Read the model definition and answer for the solid it produces. Units are mm, in the model's axes. A direction names the side the tool comes from. Coordinates: 2 decimals unless noted, no trailing zeros. Loops run counter-clockwise (first coordinate to the right, second up) from the corner with the lowest first, then second, coordinate; pieces in that order, holes last. Notation, with made-up numbers: (61, -24) - (104, -24) arc R20 ccw to (104, -17) - close; hole circle Ø8 at (16, -5). An arc over 180 degrees is marked (long way). One line per item, written item: value. Start each with the question number.
from build123d import *

# Parameters (mm, degrees)
EXTRUDE1_DEPTH                                      = 8
CBORE_FOR_M4_HEX_SOCKET_HEAD_CAP_SCREW1_D           = 4.5
CBORE_FOR_M4_HEX_SOCKET_HEAD_CAP_SCREW1_CBORE_D     = 8
CBORE_FOR_M4_HEX_SOCKET_HEAD_CAP_SCREW1_CBORE_DEPTH = 4.4
M5_TAPPED_HOLE1_D                                   = 4.2


with BuildPart() as part:
    # Sketch1 → Extrude1 (new body)
    with BuildSketch(Plane.XY):
        with BuildLine():
            Line((0, 6), (0, 14))
            ThreePointArc((0, 14), (-1.757359313, 18.242640687), (-6, 20))
            Line((-6, 20), (-7, 20))
            ThreePointArc((-7, 20), (-11.242640687, 21.757359313), (-13, 26))
            Line((-13, 26), (-13, 29))
            ThreePointArc((-13, 29), (-11.242640687, 33.242640687), (-7, 35))
            Line((-7, 35), (6, 35))
            ThreePointArc((6, 35), (10.242640687, 33.242640687), (12, 29))
            Line((12, 29), (12, 0))
            Line((12, 0), (6, 0))
            ThreePointArc((6, 0), (1.757359313, 1.757359313), (0, 6))
        make_face()
    extrude(amount=EXTRUDE1_DEPTH)

    # CBORE for M4 Hex Socket Head Cap Screw1 (through all)
    with Locations(Plane.XY.offset(8)):
        with Locations((-6.5, 27.5), (5.5, 27.5)):
            CounterBoreHole(CBORE_FOR_M4_HEX_SOCKET_HEAD_CAP_SCREW1_D / 2, CBORE_FOR_M4_HEX_SOCKET_HEAD_CAP_SCREW1_CBORE_D / 2, CBORE_FOR_M4_HEX_SOCKET_HEAD_CAP_SCREW1_CBORE_DEPTH)

    # M5 Tapped Hole1 (through all)
    with Locations(Plane(origin=(12, 0, 0), x_dir=(0, 0, -1), z_dir=(1, 0, 0))):
        with Locations((-4, 7)):
            Hole(M5_TAPPED_HOLE1_D / 2)


solid = part.part
1) Section C-C, the plane y = 27.5 is taken. Determine the outline of the cut face in (x, z), and give its area (3 significant figures).
2) Determine the mould class of faces 4 (the cylindrical face through (-7.538, 25.504, 1.775)), 5 (the cylindrical face through (-7.021, 31.466, 5.831)), 6 (the flat face through (0, 11, 4)), 7 (the flat face through (9, 0, 4)) for opening direction X: released by +X, released by -X, zero draft, split by the parting line, or undercut.
3) Straight lines are drawn through the part: L1, parallel to X at y = 26, z = 4.5; L2, parallel to Y at x = -6.5, z = 1.3; L3, parallel to Y at x = -6.5, z = 5.2. For each, find the intervals that lie inside material, in ascending order.
4) Section B-B, the plane y = 7 is taken. Determine the outline of the cut face in (x, z).
5) Section D-D, the plane z = 5.25 is taken. Determine the outline of the cut face in (x, y).
6) For faces 1 (the flat face through (12, 15, 4)), 2 (the flat face through (-6.5, 20, 3.9)), 3 (the flat face through (7.2, 25.8, 3.6)), determine the directions among +Z, -Z, +X, -X, +Y, -Y from which every point of the face is accessible in a straight line to the end or side of a thin tool.
7) Flat-ended cylindrical pins translate along their axes: P1, Ø7, axis at x = -6.5, y = 27.5, coming from the +Z side; P2, Ø1.5, axis at x = -5.5, z = 6.5, coming from the -Y side; P3, Ø4, axis at y = 8, z = 2.5, coming from the -X side. Find the tip coordinate at first contact, or state that the pin passes through.
8) Section A-A, the plane x = -6.5 is taken. Determine the outline of the cut face in (y, z).
Answer below:
1. outline: (-13, 0) - (-8.75, 0) - (-8.75, 3.6) - (-10.5, 3.6) - (-10.5, 8) - (-13, 8) - close; (-4.25, 0) - (3.25, 0) - (3.25, 3.6) - (1.5, 3.6) - (1.5, 8) - (-2.5, 8) - (-2.5, 3.6) - (-4.25, 3.6) - close; (7.75, 0) - (12, 0) - (12, 8) - (9.5, 8) - (9.5, 3.6) - (7.75, 3.6) - close
1. area: 97.2 mm2
2. face 4: undercut
2. face 5: undercut
2. face 6: released by -X
2. face 7: zero draft
3. L1: -13 to -10.21, -2.79 to 1.79, 9.21 to 12
3. L2: 20 to 25.25, 29.75 to 35
3. L3: 20 to 23.5, 31.5 to 35
4. outline: (0, 0) - (12, 0) - (12, 1.9) - (0, 1.9) - close; (0, 6.1) - (12, 6.1) - (12, 8) - (0, 8) - close
5. outline: (-13, 26) arc R6 ccw to (-7, 20) - (-6, 20) arc R6 cw to (0, 14) - (0, 8.69) - (12, 8.69) - (12, 29) arc R6 ccw to (6, 35) - (-7, 35) arc R6 ccw to (-13, 29) - close; (0.04, 5.31) arc R6 ccw to (6, 0) - (12, 0) - (12, 5.31) - close; hole circle Ø8 at (-6.5, 27.5); hole circle Ø8 at (5.5, 27.5)
6. face 1: +Z, -Z, +X, +Y, -Y
6. face 2: +Z, -Z, -X, -Y
6. face 3: +Z
7. P1: z = 3.6
7. P2: y = 19.87
7. P3: x = 0
8. outline: (20, 0) - (25.25, 0) - (25.25, 3.6) - (23.5, 3.6) - (23.5, 8) - (20, 8) - close; (29.75, 0) - (35, 0) - (35, 8) - (31.5, 8) - (31.5, 3.6) - (29.75, 3.6) - close
